Verification items for the finished model (mm, model axes). Round coordinates to 2 decimals unless told otherwise and drop trailing zeros. Write each loop counter-clockwise with the first axis right and the second up, starting at its lowest first coordinate (ties: lowest second). Pieces come first, ordered by that corner, then holes. Notation, with made-up numbers: M 21,15.5 L 80,15.5 A9 ccw 80,22.5 Z; hole C 77.5,30 d3. An arc over 180 degrees is marked long. One line per question, with ' | ' between items. Start each with the question number.
Q1. Cross-section at C-C (x = 51). Record the boundary of the cut face in (y, z) (3 decimals).
Q2. Cross-section at D-D (x = 24). Record the boundary of the cut face in (y, z) (3 decimals).
Q3. Thickness scan on line 1 along X through (y, z) = (50.8, 2.15); line 2 along Y through (x, z) = (49, 1.7); line 3 along Y through (x, z) = (6.5, 2.65). Record the ranges inside material, lowest first. Write a range as from..to.
Q4. Gauge pin test, flat end, axial feed: pin 1 (1 mm diameter, centred on y = 113.5, z = 1, fed in from +X) (3 decimals). Record the tip position at first contact, or that the pin passes through.
Q5. Cross-section at B-B (y = 0). Record the boundary of the cut face in (x, z) (1 decimal), then the cut area to 3 significant figures.
Q6. Cross-section at A-A (z = 0.75). State how many separate pieces and enclosed holes the cut face has, then the cut area to 3 significant figures.
from build123d import *

# Parameters (mm, degrees)
F0_W     = 22.225
F0_H     = 76.2
F1_DEPTH = 3.175


with BuildPart() as f1:
    # F0 (on Top) → F1 (new body)
    with BuildSketch(Plane.XY):
        with BuildLine():
            Line((-68.2625, -19.05), (68.2625, -19.05))
            Line((68.2625, -19.05), (68.2625, 19.05))
            Line((68.2625, 19.05), (68.2625, 50.8))
            ThreePointArc((68.2625, 50.8), (62.6828841816, 64.2703841816), (49.2125, 69.85))
            Line((49.2125, 69.85), (49.2125, 60.325))
            ThreePointArc((49.2125, 60.325), (55.9476920908, 57.5351920908), (58.7375, 50.8))
            ThreePointArc((58.7375, 50.8), (49.2125, 41.275), (39.6875, 50.8))
            Line((39.6875, 50.8), (-39.6875, 50.8))
            ThreePointArc((-39.6875, 50.8), (-55.9476920908, 44.0648079092), (-49.2125, 60.325))
            Line((-49.2125, 60.325), (-49.2125, 69.85))
            ThreePointArc((-49.2125, 69.85), (-62.6828841816, 64.2703841816), (-68.2625, 50.8))
            Line((-68.2625, 50.8), (-68.2625, 19.05))
            Line((-68.2625, 19.05), (-68.2625, -19.05))
        make_face()
        with BuildLine():
            Line((-45.4025, -3.302), (-53.0225, -3.302))
            ThreePointArc((-53.0225, -3.302), (-56.3245, 0), (-53.0225, 3.302))
            Line((-53.0225, 3.302), (-45.4025, 3.302))
            ThreePointArc((-45.4025, 3.302), (-42.1005, 0), (-45.4025, -3.302))
        make_face(mode=Mode.SUBTRACT)
        with BuildLine():
            Line((19.05, 18.25625), (-19.05, 18.25625))
            ThreePointArc((-19.05, 18.25625), (-19.84375, 19.05), (-19.05, 19.84375))
            Line((-19.05, 19.84375), (19.05, 19.84375))
            ThreePointArc((19.05, 19.84375), (19.84375, 19.05), (19.05, 18.25625))
        make_face(mode=Mode.SUBTRACT)
        with BuildLine():
            Line((45.4025, 3.302), (53.0225, 3.302))
            ThreePointArc((53.0225, 3.302), (56.3245, 0), (53.0225, -3.302))
            Line((53.0225, -3.302), (45.4025, -3.302))
            ThreePointArc((45.4025, -3.302), (42.1005, 0), (45.4025, 3.302))
        make_face(mode=Mode.SUBTRACT)
        with BuildLine():
            Line((49.2125, 60.325), (49.2125, 69.85))
            Line((49.2125, 69.85), (22.225, 69.85))
            Line((22.225, 69.85), (0, 69.85))
            Line((0, 69.85), (-22.225, 69.85))
            Line((-22.225, 69.85), (-49.2125, 69.85))
            Line((-49.2125, 69.85), (-49.2125, 60.325))
            ThreePointArc((-49.2125, 60.325), (-42.4773079092, 57.5351920908), (-39.6875, 50.8))
            Line((-39.6875, 50.8), (39.6875, 50.8))
            ThreePointArc((39.6875, 50.8), (42.4773079092, 57.5351920908), (49.2125, 60.325))
        make_face()
        with Locations((11.1125, 107.95)):
            Rectangle(F0_W, F0_H)
        with Locations((-11.1125, 107.95)):
            Rectangle(F0_W, F0_H)
    extrude(amount=F1_DEPTH)


solid = f1.part
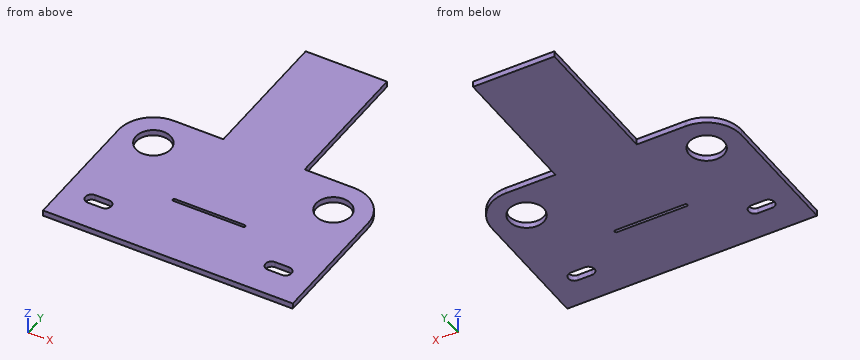
Determined:
1) outline: M -19.05,0 L -3.302,0 L -3.302,3.175 L -19.05,3.175 Z; M 3.302,0 L 41.444,0 L 41.444,3.175 L 3.302,3.175 Z; M 60.156,0 L 69.766,0 L 69.766,3.175 L 60.156,3.175 Z
2) outline: M -19.05,0 L 69.85,0 L 69.85,3.175 L -19.05,3.175 Z
3) line 1: x = -68.26..-58.74, -39.69..39.69, 58.74..68.26 | line 2: y = -19.05..-3.3, 3.3..41.28, 60.32..69.85 | line 3: y = -19.05..18.26, 19.84..146.05
4) pin 1: stops at x = 22.225
5) outline: M -68.3,0 L -56.3,0 L -56.3,3.2 L -68.3,3.2 Z; M -42.1,0 L 42.1,0 L 42.1,3.2 L -42.1,3.2 Z; M 56.3,0 L 68.3,0 L 68.3,3.2 L 56.3,3.2 Z | area: 343 mm²
6) separate pieces: 1 | enclosed holes: 5 | area: 14,600 mm²
